from build123d import *

# Parameters (mm, degrees)
SKETCH1_W           = 110
SKETCH1_H           = 80
SKETCH1_R           = 4
BOSS_EXTRUDE1_DEPTH = 5
SKETCH2_R           = 1
BOSS_EXTRUDE2_DEPTH = 15
FILLET1_R           = 5
SKETCH3_W           = 41
SKETCH3_H           = 13
CUT_EXTRUDE2_DEPTH  = 5


with BuildPart() as part:
    # Sketch1 → Boss-Extrude1 (new body)
    with BuildSketch(Plane(origin=(0, 0, 0), x_dir=(1, 0, 0), z_dir=(0, 1, 0))):
        Rectangle(SKETCH1_W, SKETCH1_H)
        with Locations(Location((-35.06, 22.32, 0), (0, 0, 270))):
            Circle(SKETCH1_R, mode=Mode.SUBTRACT)
        with Locations(Location((-35.06, 3.27, 0), (0, 0, 270))):
            Circle(SKETCH1_R, mode=Mode.SUBTRACT)
        with Locations(Location((-35.06, -6.89, 0), (0, 0, 270))):
            Circle(SKETCH1_R, mode=Mode.SUBTRACT)
        with Locations(Location((-35.06, -17.05, 0), (0, 0, 270))):
            Circle(SKETCH1_R, mode=Mode.SUBTRACT)
        with Locations(Location((-35.06, -25.95, 0), (0, 0, 270))):
            Circle(SKETCH1_R, mode=Mode.SUBTRACT)
    extrude(amount=BOSS_EXTRUDE1_DEPTH)

    # Sketch2 → Boss-Extrude2 (add)
    with BuildSketch(Plane(origin=(0, 5, 0), x_dir=(1, 0, 0), z_dir=(0, 1, 0))):
        with Locations(Location((47.1, 31.5, 0), (0, 0, 90))):
            Circle(SKETCH2_R)
        with Locations(Location((47.1, -31.5, 0), (0, 0, 90))):
            Circle(SKETCH2_R)
        with Locations(Location((-46.5, 31.5, 0), (0, 0, 90))):
            Circle(SKETCH2_R)
        with Locations(Location((-46.5, -31.5, 0), (0, 0, 90))):
            Circle(SKETCH2_R)
    extrude(amount=BOSS_EXTRUDE2_DEPTH)

    # Fillet1
    fillet1_edges = [part.edges().sort_by_distance(p)[0] for p in [
        (55, 2.5, 40),
        (-55, 2.5, 40),
        (-55, 2.5, -40),
        (55, 2.5, -40),
    ]]
    fillet(fillet1_edges, radius=FILLET1_R)

    # Sketch3 → Cut-Extrude2 (cut)
    with BuildSketch(Plane.XZ):
        with Locations((19.3, -8.18)):
            Rectangle(SKETCH3_W, SKETCH3_H)
    extrude(amount=-CUT_EXTRUDE2_DEPTH, mode=Mode.SUBTRACT)


solid = part.part
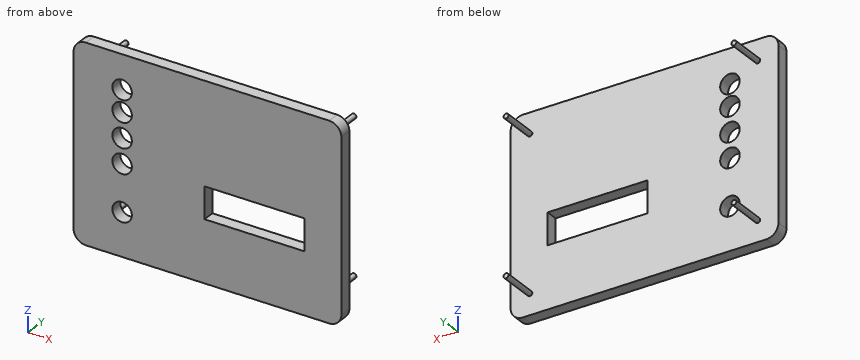
For this review, take the finished solid that the model builds, in its own axes (mm). Give positions to 0.01 mm unless a question says otherwise; leave off trailing zeros. Order: outer loops, then holes, each group sorted by start corner. A loop starts at its lowest first (then second) coordinate and runs counter-clockwise, first axis right, second up. Notation, with made-up numbers: M 70.25,88.5 L 75.25,88.5 A22 ccw 75.25,106.5 Z; hole C 14,-8.75 d2. An arc over 180 degrees is marked long. Answer in a Markdown table with one row per item. Add a question column.
(1) Consider section C-C on x = 32. State the section outline as (y, z) points.
(2) Consider section A-A on z = 6.89. State the section outline as (x, y) points, and give its area (3 significant figures).
(3) Wall thickness on probe 1 along X at (y, z) = (1.5, -22.32); probe 2 along X at (y, z) = (3.6, -3.27); probe 3 along Y at (x, z) = (-14, 36): over which ranges is each line inside the solid? List them lowest first. Write a range as [from, to].
(4) Consider section D-D on z = -3.27. State the section outline as (x, y) points.
(5) For pin 1 (24 mm diameter, centred on x = 1, z = -4.5, fed in from +Y); pin 2 (8 mm diameter, centred on y = 6, z = 13.5, fed in from +X); pin 3 (5 mm diameter, centred on x = -35.06, z = -22.32, fed in from -Y); pin 4 (5 mm diameter, centred on x = -43.5, y = 16.5, fed in from -Z), all flat-tipped, find the tip position at first contact; note any pin that passes through.
(6) Consider section B-B on y = 2. State the section outline as (x, z) points, and give its area (3 significant figures).
Evaluation:
| question | item | result |
|---|---|---|
| 1 | outline | M 0,-40 L 5,-40 L 5,-14.68 L 0,-14.68 Z; M 0,-1.68 L 5,-1.68 L 5,40 L 0,40 Z |
| 2 | outline | M -55,0 L -39.06,0 L -39.06,5 L -55,5 Z; M -31.06,0 L 55,0 L 55,5 L -31.06,5 Z |
| 2 | area | 510 mm^2 |
| 3 | probe 1 | x = [-55, -39.06], [-31.06, 55] |
| 3 | probe 2 | x = [-55, -39.06], [-31.06, -1.2], [39.8, 55] |
| 3 | probe 3 | y = [0, 5] |
| 4 | outline | M -55,0 L -39.06,0 L -39.06,5 L -55,5 Z; M -31.06,0 L -1.2,0 L -1.2,5 L -31.06,5 Z; M 39.8,0 L 55,0 L 55,5 L 39.8,5 Z |
| 5 | pin 1 | stops at y = 5 |
| 5 | pin 2 | stops at x = 55 |
| 5 | pin 3 | passes through |
| 5 | pin 4 | stops at z = -32.37 |
| 6 | outline | M -55,-35 A5 ccw -50,-40 L 50,-40 A5 ccw 55,-35 L 55,35 A5 ccw 50,40 L -50,40 A5 ccw -55,35 Z; hole C -35.06,-22.32 d8; hole C -35.06,-3.27 d8; hole C -35.06,6.89 d8; hole C -35.06,17.05 d8; hole C -35.06,25.95 d8; hole M -1.2,-14.68 L 39.8,-14.68 L 39.8,-1.68 L -1.2,-1.68 Z |
| 6 | area | 7,990 mm^2 |
